from build123d import *

# Parameters (mm, degrees)
SKETCH_W     = 10.66
SKETCH_H     = 8.5
PAD_DEPTH    = 2.54
SKETCH001_W  = 1
SKETCH001_H  = 1
POCKET_DEPTH = 6.5
SKETCH002_W  = 0.6
SKETCH002_H  = 0.6
PAD001_DEPTH = 1.9
SKETCH003_W  = 0.6
SKETCH003_H  = 0.6
PAD002_DEPTH = 4.5


with BuildPart() as part:
    # Sketch → Pad (new body)
    with BuildSketch(Plane.XY):
        with Locations((0, 4.25)):
            Rectangle(SKETCH_W, SKETCH_H)
    extrude(amount=PAD_DEPTH)

    # Sketch001 → Pocket (cut)
    with BuildSketch(Plane(origin=(0, 8.5, 0), x_dir=(-1, 0, 0), z_dir=(0, 1, 0))):
        with Locations((-3.81, 1.27)):
            Rectangle(SKETCH001_W, SKETCH001_H)
        with Locations((-1.27, 1.27)):
            Rectangle(SKETCH001_W, SKETCH001_H)
        with Locations((1.27, 1.27)):
            Rectangle(SKETCH001_W, SKETCH001_H)
        with Locations((3.81, 1.27)):
            Rectangle(SKETCH001_W, SKETCH001_H)
    extrude(amount=-POCKET_DEPTH, mode=Mode.SUBTRACT)

    # Sketch002 → Pad001 (new body)
    with BuildSketch(Plane.XZ):
        with Locations((-3.81, 1.27)):
            Rectangle(SKETCH002_W, SKETCH002_H)
        with Locations((-1.27, 1.27)):
            Rectangle(SKETCH002_W, SKETCH002_H)
        with Locations((1.27, 1.27)):
            Rectangle(SKETCH002_W, SKETCH002_H)
        with Locations((3.81, 1.27)):
            Rectangle(SKETCH002_W, SKETCH002_H)
    extrude(amount=PAD001_DEPTH)

    # Sketch003 → Pad002 (new body)
    with BuildSketch(Plane(origin=(0, 0, 0.97), x_dir=(1, 0, 0), z_dir=(0, 0, -1))):
        with Locations((-3.81, 1.6)):
            Rectangle(SKETCH003_W, SKETCH003_H)
        with Locations((-1.27, 1.6)):
            Rectangle(SKETCH003_W, SKETCH003_H)
        with Locations((1.27, 1.6)):
            Rectangle(SKETCH003_W, SKETCH003_H)
        with Locations((3.81, 1.6)):
            Rectangle(SKETCH003_W, SKETCH003_H)
    extrude(amount=PAD002_DEPTH)


solid = part.part
Could you check a few things on this model? Use its own coordinates, in mm. A direction names the side the tool comes from. Coordinates: 2 decimals unless noted, no trailing zeros. Order: outer loops, then holes, each group sorted by start corner. A loop starts at its lowest first (then second) coordinate and runs counter-clockwise, first axis right, second up. Notation, with made-up numbers: (87, 51.5) - (136, 51.5) arc R19 cw to (136, 82.5) - close; hole circle Ø7 at (0, 27.5). An arc over 180 degrees is marked (long way). Answer in a Markdown table with one row per item. Add a question column.
(1) On a 3-axis mill with a long thin cutter (end or side, diameter ignored), from which of +Z, -Z, +X, -X, +Y, -Y can I reach the whole of each face in a straight line? I mean faces 1 (the face through (1, 5, 1.77)), 2 (the face through (0, 4, 2.54)), 3 (the face through (4.11, -1.6, -0.4)), 4 (the face through (-3.51, -1.6, -0.4)). Say none if no direction works.
(2) If we section it at B-B, the plane z = -1.75: Please give me the cut outline in (x, y).
(3) I need wall thicknesses on L1, parallel to X at y = 7.25, z = 1.25; L2, parallel to X at y = -1.5, z = -2; L3, parallel to Z at x = 1, y = 5.5. Which ranges of each line are inside material? Lowest first, please.
(4) If we section it at D-D, the plane x = -3.75: Please give me the cut outline in (y, z).
(5) If we section it at C-C, the plane y = 2.75: Please give me the cut outline in (x, z).
(6) If we mould it in two halves opening along X, with no side actions, what happens to faces 5 (the face through (-4.11, -1.6, -0.4)), 6 (the face through (-4.31, 5, 1)), 7 (the face through (0, 4, 0))? For each: released by +X, released by -X, zero draft, split by the parting line, or undercut.
(7) If we section it at A-A, the plane y = -1: Please give me the cut outline in (x, z).
(8) Will these pins go through, and if not, where does the flat tip stop? pin 1 (1 mm diameter, centred on y = -1, z = -1, fed in from +X); pin 2 (0.8 mm diameter, centred on x = -1.5, y = 7, fed in from -Z); pin 3 (0.5 mm diameter, centred on x = 4, y = -0.5, fed in from +Z); pin 4 (3 mm diameter, centred on y = 5.5, z = -0.5, fed in from -X).
Results are:
| question | item | result |
|---|---|---|
| 1 | face 1 | +Y |
| 1 | face 2 | +Z, +X, -X, +Y, -Y |
| 1 | face 3 | +Z, -Z, +X, -Y |
| 1 | face 4 | +Z, -Z, -Y |
| 2 | outline | (-4.11, -1.9) - (-3.51, -1.9) - (-3.51, -1.3) - (-4.11, -1.3) - close; (-1.57, -1.9) - (-0.97, -1.9) - (-0.97, -1.3) - (-1.57, -1.3) - close; (0.97, -1.9) - (1.57, -1.9) - (1.57, -1.3) - (0.97, -1.3) - close; (3.51, -1.9) - (4.11, -1.9) - (4.11, -1.3) - (3.51, -1.3) - close |
| 3 | L1 | x = -5.33 to -4.31, -3.31 to -1.77, -0.77 to 0.77, 1.77 to 3.31, 4.31 to 5.33 |
| 3 | L2 | x = -4.11 to -3.51, -1.57 to -0.97, 0.97 to 1.57, 3.51 to 4.11 |
| 3 | L3 | z = 0 to 0.77, 1.77 to 2.54 |
| 4 | outline | (-1.9, -3.53) - (-1.3, -3.53) - (-1.3, 0.97) - (0, 0.97) - (0, 0) - (8.5, 0) - (8.5, 0.77) - (2, 0.77) - (2, 1.77) - (8.5, 1.77) - (8.5, 2.54) - (0, 2.54) - (0, 1.57) - (-1.9, 1.57) - close |
| 5 | outline | (-5.33, 0) - (5.33, 0) - (5.33, 2.54) - (-5.33, 2.54) - close; hole (-4.31, 0.77) - (-3.31, 0.77) - (-3.31, 1.77) - (-4.31, 1.77) - close; hole (-1.77, 0.77) - (-0.77, 0.77) - (-0.77, 1.77) - (-1.77, 1.77) - close; hole (0.77, 0.77) - (1.77, 0.77) - (1.77, 1.77) - (0.77, 1.77) - close; hole (3.31, 0.77) - (4.31, 0.77) - (4.31, 1.77) - (3.31, 1.77) - close |
| 6 | face 5 | released by -X |
| 6 | face 6 | undercut |
| 6 | face 7 | zero draft |
| 7 | outline | (-4.11, 0.97) - (-3.51, 0.97) - (-3.51, 1.57) - (-4.11, 1.57) - close; (-1.57, 0.97) - (-0.97, 0.97) - (-0.97, 1.57) - (-1.57, 1.57) - close; (0.97, 0.97) - (1.57, 0.97) - (1.57, 1.57) - (0.97, 1.57) - close; (3.51, 0.97) - (4.11, 0.97) - (4.11, 1.57) - (3.51, 1.57) - close |
| 8 | pin 1 | stops at x = 4.11 |
| 8 | pin 2 | stops at z = 0 |
| 8 | pin 3 | stops at z = 1.57 |
| 8 | pin 4 | stops at x = -5.33 |
